The listing builds one solid part. Answer for the finished solid, in the listing's coordinates (mm). A direction names the side the tool comes from. Round coordinates to 2 decimals unless told otherwise and drop trailing zeros. Write each loop counter-clockwise with the first axis right and the second up, starting at its lowest first coordinate (ties: lowest second). Pieces come first, ordered by that corner, then holes. Notation, with made-up numbers: M -20,-14.5 L 29,-14.5 A34 ccw 29,20.5 Z; hole C -13,50.5 d9. An arc over 180 degrees is marked long. One line per item, written item: value. Start each with the question number.
(1) For faces 4 (the flat face through (1, -3, 15)), 5 (the flat face through (-2, -2, 0)), 6 (the flat face through (1, 2.7, 2)), 7 (the flat face through (1, 5.3, 2)), 8 (the cylindrical face through (1.36, 7.44, 6.12)), determine the directions among +Z, -Z, +X, -X, +Y, -Y from which every point of the face is accessible in a straight line to the end or side of a thin tool.
(2) For a pull along Y with two mould halves and no side action, classify faces 1 (the cylindrical face through (-2.682, 2.034, 10.944)), 2 (the flat face through (4, 2, 7)), 3 (the conical face through (0.736, 2.414, 4.915)) as released by +Y, released by -Y, zero draft, split by the parting line, or undercut.
(3) Consider probe 1 along Z at (x, y) = (0, 7.65); probe 2 along Y at (x, z) = (-1.25, 2); probe 3 along Y at (x, z) = (0, 7.25). Determine where each line is inside the solid, lowest interval first.
(4) Section C-C (x = 1) is taken. State how many separate pieces and enclosed holes the cut face has, plus the area to 3 significant figures.
(5) Section D-D (y = -1.75) is taken. Determine the outline of the cut face in (x, z), plus the area to 3 significant figures.
(6) Section B-B (z = 11.5) is taken. Determine the outline of the cut face in (x, y), plus the area to 3 significant figures.
(7) Given P1, Ø3.5, axis at x = 0, z = 3.5, coming from the +Y side; P2, Ø0.8, axis at y = 4, z = 5, coming from the -X side; P3, Ø2, axis at y = 1.5, z = 8.5, coming from the -X side, each flat-ended and moving along its own axis, determine where each tip first touches the part or whether it passes through.
(8) Section A-A (y = 0) is taken. Determine the outline of the cut face in (x, z).
```python
from build123d import *

# Parameters (mm, degrees)
ESQUISSE1_R             = 8.5
BOSS_EXTRU_1_DEPTH      = 7
ESQUISSE2_W             = 6
ESQUISSE2_H             = 2.6
ENL_V_MAT_EXTRU_1_DEPTH = 14.910427743
ESQUISSE7_R             = 2.95
ENL_V_MAT_EXTRU_8_DEPTH = 21.087060672
ESQUISSE9_R             = 4.05
BOSS_EXTRU_2_DEPTH      = 8
ENL_V_MAT_EXTRU_9_DEPTH = 20.222382876


with BuildPart() as part:
    # Esquisse1 → Boss.-Extru.1 (new body)
    with BuildSketch(Plane.XY):
        Circle(ESQUISSE1_R)
    extrude(amount=BOSS_EXTRU_1_DEPTH)

    # Esquisse2 → Enlèv. mat.-Extru.1 (cut, through all)
    with BuildSketch(Plane(origin=(0, 0, 0), x_dir=(-1, 0, 0), z_dir=(0, 0, -1))):
        with Locations((0, 4)):
            Rectangle(ESQUISSE2_W, ESQUISSE2_H)
    extrude(amount=-ENL_V_MAT_EXTRU_1_DEPTH, mode=Mode.SUBTRACT)

    # Enlèv. mat.-Extru.2: read off the stored shape, not the designer's step
    # Enlèv. mat.-Extru.2 outline → Enlèv. mat.-Extru.2 (revolve, cut)
    with BuildSketch(Plane.XY.offset(3.5)):
        Polygon((0, 5.3), (1.554616831, 5.3), (1.498760014, 8.500034923), (0, 8.500034923), align=None)
        Polygon((1.6, 2.7), (0, 2.7), (0, 0.7), (1.56508987, 0.7), align=None)
    revolve(axis=Axis((0, 0, 3.5), (0, 1, 0)), mode=Mode.SUBTRACT)

    # Esquisse7 → Enlèv. mat.-Extru.8 (cut, through all)
    with BuildSketch(Plane(origin=(0, 8.3, 0), x_dir=(1, 0, 0), z_dir=(0, 1, 0))):
        with Locations((0, -3.5)):
            Circle(ESQUISSE7_R)
    extrude(amount=ENL_V_MAT_EXTRU_8_DEPTH, mode=Mode.SUBTRACT)

    # Chanfrein1: read off the stored shape, not the designer's step
    # Chanfrein1 outline → Chanfrein1 (revolve, cut)
    with BuildSketch(Plane.XY.offset(3.5)):
        Polygon((2.95, 6.747748364), (2.95, 8.3), (1.502251636, 8.3), (1.553718474, 5.351466838), align=None)
    revolve(axis=Axis((0, 0, 3.5), (0, 1, 0)), mode=Mode.SUBTRACT)

    # Esquisse9 → Boss.-Extru.2 (add)
    with BuildSketch(Plane.XY.offset(7)):
        with Locations(Location((0, -1, 0), (0, 0, 113.995098868))):
            Circle(ESQUISSE9_R)
    extrude(amount=BOSS_EXTRU_2_DEPTH)

    # Esquisse10 → Enlèv. mat.-Extru.9 (cut, through all)
    with BuildSketch(Plane(origin=(0, 0, 0), x_dir=(-1, 0, 0), z_dir=(0, 0, -1))):
        with BuildLine():
            Line((-1.549193338, 2.15), (1.549193338, 2.15))
            ThreePointArc((1.549193338, 2.15), (0, -2.65), (-1.549193338, 2.15))
        make_face()
    extrude(amount=-ENL_V_MAT_EXTRU_9_DEPTH, mode=Mode.SUBTRACT)


solid = part.part
```
Recorded:
1. face 4: +Z, +X, -X, +Y, -Y
1. face 5: -Z, +X, -X, +Y, -Y
1. face 6: -Z
1. face 7: +Z, -Z
1. face 8: +Y
2. face 1: split by the parting line
2. face 2: zero draft
2. face 3: undercut
3. probe 1: z = 0 to 0.55, 6.45 to 7
3. probe 2: y = -8.41 to -2.34, 2.15 to 2.7, 5.3 to 5.75
3. probe 3: y = -5.05 to -2.65, 2.15 to 3.05
4. separate pieces: 5
4. enclosed holes: 0
4. area: 77.2 mm2
5. outline: M -8.32,0 L -1.99,0 L -1.99,15 L -3.98,15 L -3.98,7 L -8.32,7 Z; M 1.99,0 L 8.32,0 L 8.32,7 L 3.98,7 L 3.98,15 L 1.99,15 Z
5. area: 120 mm2
6. outline: C 0,-1 d8.1; hole M -1.55,2.15 A2.65 ccw long 1.55,2.15 Z
6. area: 30.5 mm2
7. P1: stops at y = 5.55
7. P2: stops at x = -7.7
7. P3: stops at x = -3.76
8. outline: M -8.5,0 L -2.65,0 L -2.65,15 L -3.92,15 L -3.92,7 L -8.5,7 Z; M 2.65,0 L 8.5,0 L 8.5,7 L 3.92,7 L 3.92,15 L 2.65,15 Z
